Geometry check sheet. Reference: the model listing, model coordinates, mm. Coordinates: 2 decimals unless noted, no trailing zeros. Order: outer loops, then holes, each group sorted by start corner. A loop starts at its lowest first (then second) coordinate and runs counter-clockwise, first axis right, second up. Notation, with made-up numbers: M -18,89 L 13,89 A36 ccw 13,127 Z; hole C 48.25,32 d4. An arc over 180 degrees is marked long. One line per item, written item: value. Start each with the question number.
1) Sectioned sample at B-B, the plane y = -17.25. Enter the section's corners in (x, z), then the cut area to 3 significant figures.
2) Go/stop test with flat-tipped pins: P1, Ø8, axis at y = -10, z = 12, coming from the +X side; P2, Ø1.5, axis at y = -12, z = 23, coming from the -X side; P3, Ø6, axis at x = 107.5, y = -12.5, coming from the +Z side; P4, Ø3, axis at y = -16, z = 17, coming from the +X side. Record where each tip stops, or that it passes through.
3) Thickness scan on L1, parallel to Y at x = 56, z = -18; L2, parallel to Y at x = 15, z = -6; L3, parallel to X at y = -5, z = -2. Record the ranges inside material, lowest first. Write a range as from..to.
4) Sectioned sample at A-A, the plane x = 90. Enter the section's corners in (y, z), then the cut area to 3 significant figures.
```python
from build123d import *

# Parameters (mm, degrees)
EXTRUDE_1_DEPTH          = 20
CUT_EXTRUDE_1_DEPTH      = 168.622030081
CUT_EXTRUDE_1_DEPTH_BACK = 168.622030081
FILLET_1_R               = 10


with BuildPart() as part:
    # 草图3 → 凸台-拉伸1 (new body)
    with BuildSketch(Plane(origin=(0, 0, 0), x_dir=(1, 0, 0), z_dir=(0, 1, 0))):
        with BuildLine():
            Line((163.730296133, -29.825074964), (80.579718414, -29.825074964))
            Line((80.579718414, -29.825074964), (30.579718414, -25.450641788))
            ThreePointArc((30.579718414, -25.450641788), (7.258501946, 0), (30.579718414, 25.450641788))
            Line((30.579718414, 25.450641788), (80.579718414, 29.825074964))
            Line((80.579718414, 29.825074964), (163.730296133, 29.825074964))
            Line((163.730296133, 29.825074964), (163.730296133, -29.825074964))
        make_face()
    extrude(amount=-EXTRUDE_1_DEPTH)

    # 草图4 → 切除-拉伸1 (cut, two sides: drawn at the far end of the back side and taken through both)
    with BuildSketch(Plane.XY.offset(-CUT_EXTRUDE_1_DEPTH_BACK)):
        with BuildLine():
            Line((163.730296133, 0), (159.58071917, 0))
            add(Edge.make_bspline(
                [(159.58071917, 0), (148.122104631, -7.824360885), (148.302724928, -20)],
                knots=[0, 0, 0, 1, 1, 1], degree=2))
            Line((148.302724928, -20), (203.221653408, -20))
            Line((203.221653408, -20), (203.221653408, 0))
            Line((203.221653408, 0), (163.730296133, 0))
        make_face()
    extrude(amount=CUT_EXTRUDE_1_DEPTH + CUT_EXTRUDE_1_DEPTH_BACK, mode=Mode.SUBTRACT)

    # 圆角1
    # the kernel refuses this fillet: 10 mm, written as the material it takes off along each edge
    with BuildSketch(Plane(origin=(55.579718414, -20, -29.825074964), x_dir=(0, 0, 1), z_dir=(1, 0, 0))) as fillet_1_piece_1_section:
        with BuildLine():
            CenterArc((FILLET_1_R, -FILLET_1_R), FILLET_1_R, 90, 90)
            Line((0, -FILLET_1_R), (-FILLET_1_R * 0.02, -FILLET_1_R))
            Line((-FILLET_1_R * 0.02, -FILLET_1_R), (-FILLET_1_R * 0.02, FILLET_1_R * 0.02))
            Line((-FILLET_1_R * 0.02, FILLET_1_R * 0.02), (FILLET_1_R, FILLET_1_R * 0.02))
            Line((FILLET_1_R, FILLET_1_R * 0.02), (FILLET_1_R, 0))
        make_face()
    fillet_1_piece_1 = extrude(amount=117.723006514, mode=Mode.PRIVATE)
    fillet_1_piece_1 = split(fillet_1_piece_1, bisect_by=Plane(origin=(118.163125223, -17.857550266, -33.113196996), z_dir=(0.08715574274764791, 0, 0.9961946980917464)), keep=Keep.TOP, mode=Mode.PRIVATE)
    add(fillet_1_piece_1, mode=Mode.SUBTRACT)
    with BuildSketch(Plane(origin=(173.302724928, -20, 29.825074964), x_dir=(0, 1, 0), z_dir=(-1, 0, 0))) as fillet_1_piece_2_section:
        with BuildLine():
            CenterArc((FILLET_1_R, FILLET_1_R), FILLET_1_R, 180, 90)
            Line((0, FILLET_1_R), (-FILLET_1_R * 0.02, FILLET_1_R))
            Line((-FILLET_1_R * 0.02, FILLET_1_R), (-FILLET_1_R * 0.02, -FILLET_1_R * 0.02))
            Line((-FILLET_1_R * 0.02, -FILLET_1_R * 0.02), (FILLET_1_R, -FILLET_1_R * 0.02))
            Line((FILLET_1_R, -FILLET_1_R * 0.02), (FILLET_1_R, 0))
        make_face()
    fillet_1_piece_2 = extrude(amount=117.723006514, mode=Mode.PRIVATE)
    fillet_1_piece_2 = split(fillet_1_piece_2, bisect_by=Plane(origin=(118.163125223, -17.857550266, 33.113196996), z_dir=(0.08715574274764758, 0, -0.9961946980917465)), keep=Keep.TOP, mode=Mode.PRIVATE)
    add(fillet_1_piece_2, mode=Mode.SUBTRACT)
    with BuildSketch(Plane(origin=(105.484585867, -20, 32.003968533), x_dir=(0, 1, 0), z_dir=(-0.9961946980917465, 0, -0.08715574274764758))) as fillet_1_piece_3_section:
        with BuildLine():
            CenterArc((FILLET_1_R, FILLET_1_R), FILLET_1_R, 180, 90)
            Line((0, FILLET_1_R), (-FILLET_1_R * 0.02, FILLET_1_R))
            Line((-FILLET_1_R * 0.02, FILLET_1_R), (-FILLET_1_R * 0.02, -FILLET_1_R * 0.02))
            Line((-FILLET_1_R * 0.02, -FILLET_1_R * 0.02), (FILLET_1_R, -FILLET_1_R * 0.02))
            Line((FILLET_1_R, -FILLET_1_R * 0.02), (FILLET_1_R, 0))
        make_face()
    fillet_1_piece_3 = extrude(amount=75.190991877, mode=Mode.PRIVATE)
    fillet_1_piece_3 = split(fillet_1_piece_3, bisect_by=Plane(origin=(64.333848785, -17.936020538, 29.825074964), z_dir=(0, 0, -1)), keep=Keep.TOP, mode=Mode.PRIVATE)
    add(fillet_1_piece_3, mode=Mode.SUBTRACT)
    with BuildSketch(Plane(origin=(148.302724928, -20, 0), x_dir=(-1, 0, 0), z_dir=(0, 0, -1))) as fillet_1_piece_4:
        with BuildLine():
            CenterArc((8.573839583, 10), FILLET_1_R, 197.276402176, 72.723597824)
            Line((-0.974992369, 7.030183787), (-1.165969008, 6.970787462))
            ThreePointArc((-1.165969008, 6.970787462), (-0.405650645, 3.526203376), (-0.199977997, 0.002966586))
            Line((-0.199977997, 0.002966586), (0, -0.2))
            Line((0, -0.2), (8.573839583, -0.2))
            Line((8.573839583, -0.2), (8.573839583, 0))
        make_face()
    extrude(amount=29.825074964, mode=Mode.SUBTRACT)
    with BuildSketch(Plane(origin=(32.80636105, -20, 0), x_dir=(-0.08715574274764748, 0, 0.9961946980917464), z_dir=(0.9961946980917464, 0, 0.08715574274764748))) as fillet_1_piece_5:
        with BuildLine():
            CenterArc((25.547859105 - FILLET_1_R, -FILLET_1_R), FILLET_1_R, 0, 90)
            Line((25.547859105, -FILLET_1_R), (25.547859105 + FILLET_1_R * 0.02, -FILLET_1_R))
            Line((25.547859105 + FILLET_1_R * 0.02, -FILLET_1_R), (25.547859105 + FILLET_1_R * 0.02, FILLET_1_R * 0.02))
            Line((25.547859105 + FILLET_1_R * 0.02, FILLET_1_R * 0.02), (25.547859105 - FILLET_1_R, FILLET_1_R * 0.02))
            Line((25.547859105 - FILLET_1_R, FILLET_1_R * 0.02), (25.547859105 - FILLET_1_R, 0))
        make_face()
    revolve(axis=Axis((32.80636105, -20, 0), (0, -1, 0)), revolution_arc=170, mode=Mode.SUBTRACT)
    with BuildSketch(Plane(origin=(30.579718414, -20, -25.450641788), x_dir=(0.0871557427476479, 0, 0.9961946980917464), z_dir=(0.9961946980917464, 0, -0.08715574274764791))) as fillet_1_piece_6_section:
        with BuildLine():
            CenterArc((FILLET_1_R, -FILLET_1_R), FILLET_1_R, 90, 90)
            Line((0, -FILLET_1_R), (-FILLET_1_R * 0.02, -FILLET_1_R))
            Line((-FILLET_1_R * 0.02, -FILLET_1_R), (-FILLET_1_R * 0.02, FILLET_1_R * 0.02))
            Line((-FILLET_1_R * 0.02, FILLET_1_R * 0.02), (FILLET_1_R, FILLET_1_R * 0.02))
            Line((FILLET_1_R, FILLET_1_R * 0.02), (FILLET_1_R, 0))
        make_face()
    fillet_1_piece_6 = extrude(amount=75.190991877, mode=Mode.PRIVATE)
    fillet_1_piece_6 = split(fillet_1_piece_6, bisect_by=Plane(origin=(64.333848785, -17.936020538, -29.825074964), z_dir=(0, 0, 1)), keep=Keep.TOP, mode=Mode.PRIVATE)
    add(fillet_1_piece_6, mode=Mode.SUBTRACT)
    with BuildSketch(Plane(origin=(148.302724928, -20, 0), x_dir=(-1, 0, 0), z_dir=(0, 0, 1))) as fillet_1_piece_7:
        with BuildLine():
            CenterArc((8.573839583, -10), FILLET_1_R, 90, 72.723597824)
            Line((-0.974992369, -7.030183787), (-1.165969008, -6.970787462))
            ThreePointArc((-1.165969008, -6.970787462), (-0.405650645, -3.526203376), (-0.199977997, -0.002966586))
            Line((-0.199977997, -0.002966586), (0, 0.2))
            Line((0, 0.2), (8.573839583, 0.2))
            Line((8.573839583, 0.2), (8.573839583, 0))
        make_face()
    extrude(amount=29.825074964, mode=Mode.SUBTRACT)
    with BuildSketch(Plane(origin=(55.579718414, -20, -29.825074964), x_dir=(0, 0, 1), z_dir=(1, 0, 0))) as fillet_1_piece_8a_section:
        with BuildLine():
            CenterArc((FILLET_1_R, -FILLET_1_R), FILLET_1_R, 90, 90)
            Line((0, -FILLET_1_R), (-FILLET_1_R * 0.02, -FILLET_1_R))
            Line((-FILLET_1_R * 0.02, -FILLET_1_R), (-FILLET_1_R * 0.02, FILLET_1_R * 0.02))
            Line((-FILLET_1_R * 0.02, FILLET_1_R * 0.02), (FILLET_1_R, FILLET_1_R * 0.02))
            Line((FILLET_1_R, FILLET_1_R * 0.02), (FILLET_1_R, 0))
        make_face()
    fillet_1_piece_8a = extrude(amount=117.723006514, mode=Mode.PRIVATE)
    fillet_1_piece_8a = split(fillet_1_piece_8a, bisect_by=Plane(origin=(65.506587176, -16.325384108, -28.506346857), z_dir=(-0.08715574274764791, 0, -0.9961946980917464)), keep=Keep.TOP, mode=Mode.PRIVATE)
    with BuildSketch(Plane(origin=(30.579718414, -20, -25.450641788), x_dir=(0.0871557427476479, 0, 0.9961946980917464), z_dir=(0.9961946980917464, 0, -0.08715574274764791))) as fillet_1_piece_8b_section:
        with BuildLine():
            CenterArc((FILLET_1_R, -FILLET_1_R), FILLET_1_R, 90, 90)
            Line((0, -FILLET_1_R), (-FILLET_1_R * 0.02, -FILLET_1_R))
            Line((-FILLET_1_R * 0.02, -FILLET_1_R), (-FILLET_1_R * 0.02, FILLET_1_R * 0.02))
            Line((-FILLET_1_R * 0.02, FILLET_1_R * 0.02), (FILLET_1_R, FILLET_1_R * 0.02))
            Line((FILLET_1_R, FILLET_1_R * 0.02), (FILLET_1_R, 0))
        make_face()
    fillet_1_piece_8b = extrude(amount=75.190991877, mode=Mode.PRIVATE)
    fillet_1_piece_8b = split(fillet_1_piece_8b, bisect_by=Plane(origin=(95.710426565, -16.325384108, -29.825074964), z_dir=(0, 0, -1)), keep=Keep.TOP, mode=Mode.PRIVATE)
    fillet_1_piece_8 = fillet_1_piece_8a & fillet_1_piece_8b
    add(fillet_1_piece_8, mode=Mode.SUBTRACT)
    with BuildSketch(Plane(origin=(173.302724928, -20, 29.825074964), x_dir=(0, 1, 0), z_dir=(-1, 0, 0))) as fillet_1_piece_9a_section:
        with BuildLine():
            CenterArc((FILLET_1_R, FILLET_1_R), FILLET_1_R, 180, 90)
            Line((0, FILLET_1_R), (-FILLET_1_R * 0.02, FILLET_1_R))
            Line((-FILLET_1_R * 0.02, FILLET_1_R), (-FILLET_1_R * 0.02, -FILLET_1_R * 0.02))
            Line((-FILLET_1_R * 0.02, -FILLET_1_R * 0.02), (FILLET_1_R, -FILLET_1_R * 0.02))
            Line((FILLET_1_R, -FILLET_1_R * 0.02), (FILLET_1_R, 0))
        make_face()
    fillet_1_piece_9a = extrude(amount=117.723006514, mode=Mode.PRIVATE)
    fillet_1_piece_9a = split(fillet_1_piece_9a, bisect_by=Plane(origin=(65.506587176, -16.325384108, 28.506346857), z_dir=(-0.08715574274764758, 0, 0.9961946980917465)), keep=Keep.TOP, mode=Mode.PRIVATE)
    with BuildSketch(Plane(origin=(105.484585867, -20, 32.003968533), x_dir=(0, 1, 0), z_dir=(-0.9961946980917465, 0, -0.08715574274764758))) as fillet_1_piece_9b_section:
        with BuildLine():
            CenterArc((FILLET_1_R, FILLET_1_R), FILLET_1_R, 180, 90)
            Line((0, FILLET_1_R), (-FILLET_1_R * 0.02, FILLET_1_R))
            Line((-FILLET_1_R * 0.02, FILLET_1_R), (-FILLET_1_R * 0.02, -FILLET_1_R * 0.02))
            Line((-FILLET_1_R * 0.02, -FILLET_1_R * 0.02), (FILLET_1_R, -FILLET_1_R * 0.02))
            Line((FILLET_1_R, -FILLET_1_R * 0.02), (FILLET_1_R, 0))
        make_face()
    fillet_1_piece_9b = extrude(amount=75.190991877, mode=Mode.PRIVATE)
    fillet_1_piece_9b = split(fillet_1_piece_9b, bisect_by=Plane(origin=(95.710426565, -16.325384108, 29.825074964), z_dir=(0, 0, 1)), keep=Keep.TOP, mode=Mode.PRIVATE)
    fillet_1_piece_9 = fillet_1_piece_9a & fillet_1_piece_9b
    add(fillet_1_piece_9, mode=Mode.SUBTRACT)


solid = part.part
```
Final values:
1. outline: M 30.85,-22.35 L 80.72,-26.71 L 146.62,-26.71 L 146.62,26.71 L 80.72,26.71 L 30.85,22.35 A22.44 ccw Z
1. area: 6,670 mm^2
2. P1: stops at x = 152.99
2. P2: stops at x = 20.63
2. P3: stops at z = 29.83
2. P4: stops at x = 148.66
3. L1: y = -19.99..0
3. L2: y = -19.46..0
3. L3: x = 7.34..153.83
4. outline: M -20,-19.83 A10 ccw -10,-29.83 L 0,-29.83 L 0,29.83 L -10,29.83 A10 ccw -20,19.83 Z
4. area: 1,150 mm^2
